The figure shows three views and two pictorial views of one solid part (mm, origin at its lowest corner). Answer the questions. Coordinates: 2 decimals unless noted, no trailing zeros. Order: outer loops, then holes, each group sorted by start corner. A loop starts at its lowest first (then second) coordinate and runs counter-clockwise, first axis right, second up. Notation, with made-up numbers: (-22, 55) - (-12, 55) arc R30 ccw to (-12, 79) - close; hole circle Ø9 at (57, 36.5). An arc over 180 degrees is marked (long way). Answer as a JSON object with one key per item and string values. Group by question number.
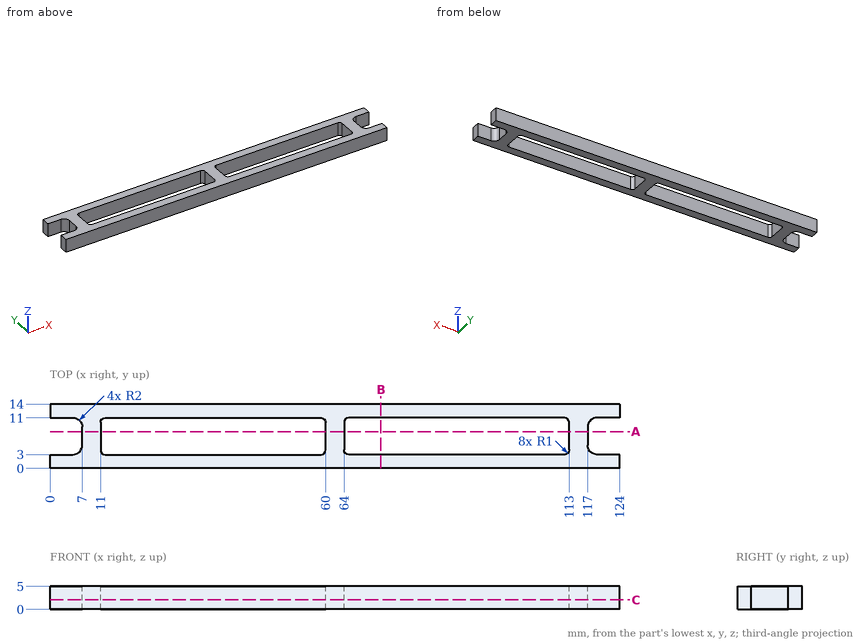
1. A cutting plane is placed at B-B on x = 72. Write down the section's boundary in (y, z), and give its area (3 significant figures).
2. A cutting plane is placed at A-A on y = 8. Write down the section's boundary in (x, z), and give its area (3 significant figures).
3. A cutting plane is placed at C-C on z = 2.05. State how many separate pieces and enclosed holes the cut face has, and give its area (3 significant figures).
4. Straight lines are drawn through the part: L1, parallel to X at y = 4.75, z = 4.6; L2, parallel to Y at x = 51, z = 1.95; L3, parallel to X at y = 10, z = 1.45. For each, find the intervals that lie inside material, in ascending order.
5. Given pin 1 (1.5 mm diameter, centred on x = 84.5, y = 10.5, fed in from +Z); pin 2 (1.2 mm diameter, centred on y = 7.5, z = 3, fed in from -X); pin 3 (1.5 mm diameter, centred on y = 7.5, z = 2, fed in from +X), each flat-ended and moving along its own axis, determine where each tip first touches the part or whether it passes through.
Derived:
{
 "1": {"outline": "(0, 0) - (3, 0) - (3, 5) - (0, 5) - close; (11, 0) - (14, 0) - (14, 5) - (11, 5) - close", "area": "30.0 mm2"},
 "2": {"outline": "(7, 0) - (11, 0) - (11, 5) - (7, 5) - close; (60, 0) - (64, 0) - (64, 5) - (60, 5) - close; (113, 0) - (117, 0) - (117, 5) - (113, 5) - close", "area": "60.0 mm2"},
 "3": {"separate pieces": "1", "enclosed holes": "2", "area": "845 mm2"},
 "4": {"L1": "x = 6.98 to 11, 60 to 64, 113 to 117.02", "L2": "y = 0 to 3, 11 to 14", "L3": "x = 6.73 to 11, 60 to 64, 113 to 117.27"},
 "5": {"pin 1": "stops at z = 5", "pin 2": "stops at x = 7", "pin 3": "stops at x = 117"}
}
